Verification items for this drawing (mm, ordinates from the low corner). Give positions to 0.01 mm unless a question says otherwise; leave off trailing zeros. Loops run counter-clockwise (first coordinate to the right, second up) from the corner with the lowest first, then second, coordinate; pieces in that order, holes last. Notation, with made-up numbers: (-39, 82.5) - (-1, 82.5) arc R10 ccw to (-1, 97.5) - close; hole circle Ø8 at (-33, -12.75). An arc over 180 degrees is marked (long way). One line per question, with ' | ' between items. Start each with the question number.
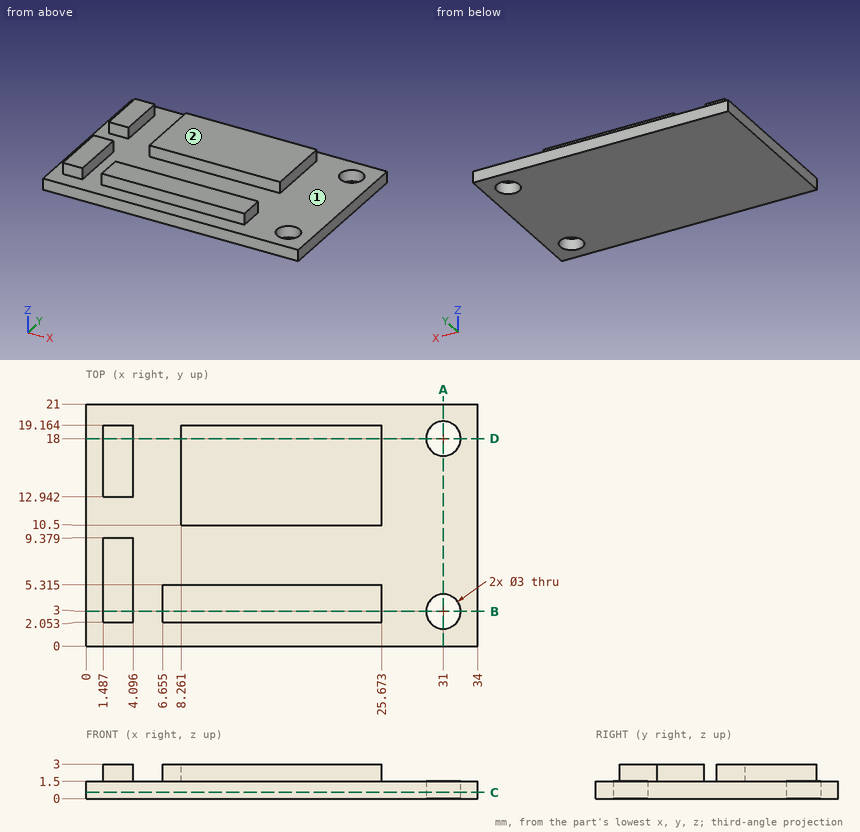
(1) Section check C-C, the plane z = 0.55. Record the boundary of the cut face in (x, y).
(2) Section check A-A, the plane x = 31. Record the boundary of the cut face in (y, z), and give its area (3 significant figures).
(3) Depth check by flat-ended pin: pin 1 Ø0.8 at (y, z) = (14.5, 2.5) entering from -X; pin 2 Ø2.5 at (x, y) = (31, 3) entering from -Z; pin 3 Ø1.2 at (x, z) = (19.5, 2.5) entering from +Y; pin 4 Ø1.6 at (y, z) = (16.5, 2.5) entering from +X. Enter the tip coordinate at first touch or a pass-through.
(4) Material ranges on line 1 (Y direction, x = 31, z = 0.9); line 2 (X direction, y = 3.5, z = 1.75) (1 decimal); line 3 (X direction, y = 18.75, z = 2.1), recorded low to high.
(5) Section check D-D, the plane y = 18. Record the boundary of the cut face in (x, z).
(6) Mould release check, pull along Y, two halves, no side actions. Record for the marked faces 1 and 2: pulls with the +Y half, pulls with the -Y half, needs draft (parallel to the pull), parting line crosses it, or undercut.
(7) Section check B-B, the plane y = 3. Record the boundary of the cut face in (x, z) (1 decimal).
Numbers:
1) outline: (0, 0) - (34, 0) - (34, 21) - (0, 21) - close; hole circle Ø3 at (31, 3); hole circle Ø3 at (31, 18)
2) outline: (0, 0) - (1.5, 0) - (1.5, 1.5) - (0, 1.5) - close; (4.5, 0) - (16.5, 0) - (16.5, 1.5) - (4.5, 1.5) - close; (19.5, 0) - (21, 0) - (21, 1.5) - (19.5, 1.5) - close | area: 22.5 mm^2
3) pin 1: x = 1.49 | pin 2: through | pin 3: y = 19.16 | pin 4: x = 25.67
4) line 1: 0 to 1.5, 4.5 to 16.5, 19.5 to 21 | line 2: 1.5 to 4.1, 6.7 to 25.7 | line 3: 1.49 to 4.1, 8.26 to 25.67
5) outline: (0, 0) - (29.5, 0) - (29.5, 1.5) - (25.67, 1.5) - (25.67, 3) - (8.26, 3) - (8.26, 1.5) - (4.1, 1.5) - (4.1, 3) - (1.49, 3) - (1.49, 1.5) - (0, 1.5) - close; (32.5, 0) - (34, 0) - (34, 1.5) - (32.5, 1.5) - close
6) face 1: undercut | face 2: needs draft
7) outline: (0, 0) - (29.5, 0) - (29.5, 1.5) - (25.7, 1.5) - (25.7, 3) - (6.7, 3) - (6.7, 1.5) - (4.1, 1.5) - (4.1, 3) - (1.5, 3) - (1.5, 1.5) - (0, 1.5) - close; (32.5, 0) - (34, 0) - (34, 1.5) - (32.5, 1.5) - close
